Geometry check sheet. Reference: the model listing, model coordinates, mm. Face numbers are marked on the shaded views. Round coordinates to 2 decimals unless told otherwise and drop trailing zeros. Order: outer loops, then holes, each group sorted by start corner. A loop starts at its lowest first (then second) coordinate and runs counter-clockwise, first axis right, second up. Notation, with made-up numbers: (41.5, -18.75) -> (87.5, -18.75) arc R16 cw to (87.5, -3.75) -> close; hole circle Ø5 at (75, 29.5). An arc over 180 degrees is marked (long way). Answer as a JSON object with one key per item and string values. Group by question number.
from build123d import *

# Parameters (mm, degrees)
F0_R     = 50.8
F0_R_2   = 31.75
F1_DEPTH = 76.2
F2_SIZE  = 5.08
F3_SIZE  = 5.08


with BuildPart() as f1:
    # F0 (on Front) → F1 (new body)
    with BuildSketch(Plane.XZ):
        Circle(F0_R)
        Circle(F0_R_2, mode=Mode.SUBTRACT)
    extrude(amount=F1_DEPTH)

    # F2
    f2_edges = [f1.edges().sort_by_distance(p)[0] for p in [
        (-31.75, -76.2, 0),
        (-31.75, 0, 0),
    ]]
    chamfer(f2_edges, length=F2_SIZE)

    # F3
    f3_edges = [f1.edges().sort_by_distance(p)[0] for p in [
        (-50.8, -76.2, 0),
        (-50.8, 0, 0),
    ]]
    chamfer(f3_edges, length=F3_SIZE)


solid = f1.part
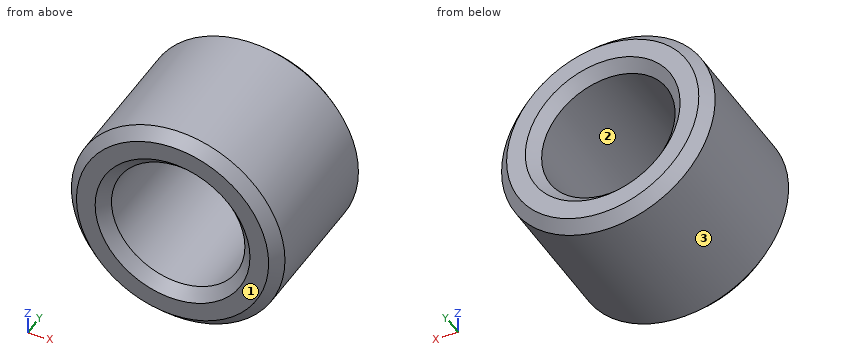
Item 1: Sectioned sample at C-C, the plane y = -65.5. Enter the section's corners in (x, z), then the cut area to 3 significant figures.
Item 2: Thickness scan on L1, parallel to Z at x = 0, y = -52; L2, parallel to X at y = -61, z = 26; L3, parallel to Z at x = -21.5, y = -64. Record the ranges inside material, lowest first.
Item 3: Depth check by flat-ended pin: pin 1 Ø1 at (x, z) = (23, 28) entering from -Y; pin 2 Ø4 at (x, y) = (4.5, -23.5) entering from -Z; pin 3 Ø1.5 at (y, z) = (-68, 5.5) entering from +X. Enter the tip coordinate at first touch or a pass-through.
Item 4: Sectioned sample at B-B, the plane z = 0. Enter the section's corners in (x, y), then the cut area to 3 significant figures.
Item 5: Mould release check, pull along Z, two halves, no side actions. Record for the marked faces 1, 2 and 3: pulls with the +Z half, pulls with the -Z half, needs draft (parallel to the pull), parting line crosses it, or undercut.
Item 6: Sectioned sample at A-A, the plane x = 0. Enter the section's corners in (y, z).
Result:
{
 "1": {"outline": "circle Ø101.6 at (0, 0); hole circle Ø63.5 at (0, 0)", "area": "4,940 mm2"},
 "2": {"L1": "z = -50.8 to -31.75, 31.75 to 50.8", "L2": "x = -43.64 to -18.22, 18.22 to 43.64", "L3": "z = -46.03 to -23.36, 23.36 to 46.03"},
 "3": {"pin 1": "stops at y = -76.11", "pin 2": "stops at z = -50.74", "pin 3": "stops at x = 50.58"},
 "4": {"outline": "(-50.8, -71.12) -> (-45.72, -76.2) -> (-36.83, -76.2) -> (-31.75, -71.12) -> (-31.75, -5.08) -> (-36.83, 0) -> (-45.72, 0) -> (-50.8, -5.08) -> close; (31.75, -71.12) -> (36.83, -76.2) -> (45.72, -76.2) -> (50.8, -71.12) -> (50.8, -5.08) -> (45.72, 0) -> (36.83, 0) -> (31.75, -5.08) -> close", "area": "2,800 mm2"},
 "5": {"face 1": "needs draft", "face 2": "undercut", "face 3": "parting line crosses it"},
 "6": {"outline": "(-76.2, -45.72) -> (-71.12, -50.8) -> (-5.08, -50.8) -> (0, -45.72) -> (0, -36.83) -> (-5.08, -31.75) -> (-71.12, -31.75) -> (-76.2, -36.83) -> close; (-76.2, 36.83) -> (-71.12, 31.75) -> (-5.08, 31.75) -> (0, 36.83) -> (0, 45.72) -> (-5.08, 50.8) -> (-71.12, 50.8) -> (-76.2, 45.72) -> close"}
}
